from build123d import *

# Parameters (mm, degrees)
F0_R     = 1.651
F1_DEPTH = 3.302


with BuildPart() as f1:
    # F0 (on Front) → F1 (new body)
    with BuildSketch(Plane.XZ):
        with BuildLine():
            Line((52.929746, 6.35), (-35.970254, 6.35))
            ThreePointArc((-35.970254, 6.35), (-34.896008, 4.771231), (-34.518209, 2.899391))
            ThreePointArc((-34.518209, 2.899391), (-34.766614, 1.371027), (-35.486256, 0))
            Line((-35.486256, 0), (52.641847, 0))
            ThreePointArc((52.641847, 0), (51.592679, 3.229094), (52.929746, 6.35))
        make_face()
        with BuildLine():
            ThreePointArc((-34.518209, 2.899391), (-34.896008, 4.771231), (-35.970254, 6.35))
            ThreePointArc((-35.970254, 6.35), (-44.156252, 2.532616), (-35.486256, 0))
            ThreePointArc((-35.486256, 0), (-34.766614, 1.371027), (-34.518209, 2.899391))
        make_face()
        with Locations((-39.344209, 2.899391)):
            Circle(F0_R, mode=Mode.SUBTRACT)
        with BuildLine():
            ThreePointArc((61.239726, 3.010515), (58.213252, 7.488459), (52.929746, 6.35))
            ThreePointArc((52.929746, 6.35), (51.592679, 3.229094), (52.641847, 0))
            ThreePointArc((52.641847, 0), (58.008591, -1.544337), (61.239726, 3.010515))
        make_face()
        with Locations((56.413726, 3.010515)):
            Circle(F0_R, mode=Mode.SUBTRACT)
    extrude(amount=F1_DEPTH)


solid = f1.part
The listing builds one solid part. Answer for the finished solid, in the listing's coordinates (mm). Give positions to 0.01 mm unless a question says otherwise; leave off trailing zeros. Order: outer loops, then holes, each group sorted by start corner. A loop starts at its lowest first (then second) coordinate and runs counter-clockwise, first axis right, second up. Notation, with made-up numbers: (-31.5, 27.5) -> (27.5, 27.5) arc R23 ccw to (27.5, 65.5) -> close; hole circle Ø11 at (-29.75, 28.25). An arc over 180 degrees is marked (long way). Put each result on its own line as item: value.
Item 1: Straight lines are drawn through the part: line 1 (X direction, y = -2.95, z = 2); line 2 (X direction, y = -1.45, z = 1.75); line 3 (Z direction, x = -16.5, y = -2.3). For each, find the intervals that lie inside material, in ascending order.
Established:
line 1: x = -44.09 to -40.73, -37.96 to 55.11, 57.72 to 61.13
line 2: x = -44.03 to -40.53, -38.16 to 55.35, 57.48 to 61.07
line 3: z = 0 to 6.35
Item 2: A cutting plane is placed at A-A on y = -1.9. Give the vertices of the cut face in (x, z).
Established:
outline: (-35.97, 6.35) arc R4.83 ccw (long way) to (-35.49, 0) -> (52.64, 0) arc R4.83 ccw (long way) to (52.93, 6.35) -> close; hole circle Ø3.3 at (-39.34, 2.9); hole circle Ø3.3 at (56.41, 3.01)
Item 3: For a pull along Z with two mould halves and no side action, classify faces 1 (the face through (-37.77, -1.63, 3.4)), 2 (the face through (9, -2, 6.35)), 3 (the face through (8, -2, 0)) as released by +Z, released by -Z, zero draft, split by the parting line, or undercut.
Established:
face 1: undercut
face 2: released by +Z
face 3: released by -Z
Item 4: Given P1, Ø1, axis at y = -1, z = 5.5, coming from the +X side; P2, Ø1, axis at x = 29, y = -1.5, coming from the +Z side, each flat-ended and moving along its own axis, determine where each tip first touches the part or whether it passes through.
Established:
P1: stops at x = 60.81
P2: stops at z = 6.35
Item 5: A cutting plane is placed at B-B on x = -16.5. Give the vertices of the cut face in (y, z), plus the area to 3 significant figures.
Established:
outline: (-3.3, 0) -> (0, 0) -> (0, 6.35) -> (-3.3, 6.35) -> close
area: 21.0 mm^2
